Part model, mm, in its own coordinate system. Face numbers are marked on the shaded views. A direction names the side the tool comes from. Coordinates: 2 decimals unless noted, no trailing zeros. Write each loop counter-clockwise with the first axis right and the second up, starting at its lowest first coordinate (ties: lowest second). Pieces come first, ordered by that corner, then holes. Notation, with made-up numbers: (-29, 23) -> (2, 23) arc R34 ccw to (2, 57) -> close; hole circle Ø10 at (81, 79). An arc over 180 degrees is marked (long way). One line per question, with ' | ' between items. Start each with the question number.
Item 1: Pin check, flat tips, straight feed: pin 1 (4 mm diameter, centred on x = 27.5, z = 75.5, fed in from +Y); pin 2 (6 mm diameter, centred on x = 32.5, y = 32.5, fed in from -Z); pin 3 (1.5 mm diameter, centred on x = 27.5, z = 65, fed in from -Y). Stop position of each tip, or through.
Item 2: Saw through at C-C (z = 69). List the corners of the cut face in (x, y).
Item 3: 3-axis set-ups, long thin cutter, end or side, ignore diameter. For the marked faces 1, 2 and 3: which of +Z, -Z, +X, -X, +Y, -Y reach the whole face in a straight line?
Item 4: Saw through at A-A (y = 32.5). List the corners of the cut face in (x, z).
Item 5: Saw through at B-B (y = 3.5). List the corners of the cut face in (x, z).
Item 6: Probe probe 1 along Y at (x, z) = (-32.5, 7.5); probe 2 along Z at (x, y) = (12, -6.5). List the from-to ranges inside material, lowest first. Write a range as [from, to].
Item 7: Saw through at D-D (x = 0). List the corners of the cut face in (y, z).
from build123d import *

# Parameters (mm, degrees)
SKETCH_1_W          = 80
SKETCH_1_H          = 80
SKETCH_1_R          = 2.7
EXTRUDE_1_DEPTH     = 130
SKETCH_2_R          = 12.5
EXTRUDE_2_DEPTH     = 140
SKETCH_3_W          = 15
SKETCH_3_H          = 15
CUT_EXTRUDE_1_DEPTH = 120
FILLET_1_R          = 2
FILLET_3_R          = 10


with BuildPart() as part:
    # 草图1 → 凸台-拉伸1 (new body)
    with BuildSketch(Plane.XY):
        Rectangle(SKETCH_1_W, SKETCH_1_H)
        with Locations((-32.5, 32.5)):
            Circle(SKETCH_1_R, mode=Mode.SUBTRACT)
        with Locations((32.5, 32.5)):
            Circle(SKETCH_1_R, mode=Mode.SUBTRACT)
        with Locations((32.5, -32.5)):
            Circle(SKETCH_1_R, mode=Mode.SUBTRACT)
        with Locations((-32.5, -32.5)):
            Circle(SKETCH_1_R, mode=Mode.SUBTRACT)
    extrude(amount=EXTRUDE_1_DEPTH)

    # 草图2 → 凸台-拉伸2 (add)
    with BuildSketch(Plane(origin=(0, 0, 0), x_dir=(-1, 0, 0), z_dir=(0, 0, -1))):
        Circle(SKETCH_2_R)
    extrude(amount=EXTRUDE_2_DEPTH)

    # 草图3 → 切除-拉伸1 (cut)
    with BuildSketch(Plane.XY.offset(130)):
        with Locations((-32.5, 32.5)):
            Rectangle(SKETCH_3_W, SKETCH_3_H)
        with Locations((32.5, 32.5)):
            Rectangle(SKETCH_3_W, SKETCH_3_H)
        with Locations((32.5, -32.5)):
            Rectangle(SKETCH_3_W, SKETCH_3_H)
        with Locations((-32.5, -32.5)):
            Rectangle(SKETCH_3_W, SKETCH_3_H)
    extrude(amount=-CUT_EXTRUDE_1_DEPTH, mode=Mode.SUBTRACT)

    # 圆角1
    fillet_1_edges = [part.edges().sort_by_distance(p)[0] for p in [
        (40, -40, 5),
        (-40, -40, 5),
        (-40, 40, 5),
        (40, 40, 5),
    ]]
    fillet(fillet_1_edges, radius=FILLET_1_R)

    # 圆角3
    fillet_3_edges = [part.edges().sort_by_distance(p)[0] for p in [
        (-25, -40, 70),
        (-40, -25, 70),
        (40, -25, 70),
        (25, -40, 70),
        (25, 40, 70),
        (40, 25, 70),
        (-40, 25, 70),
        (-25, 40, 70),
    ]]
    fillet(fillet_3_edges, radius=FILLET_3_R)


solid = part.part
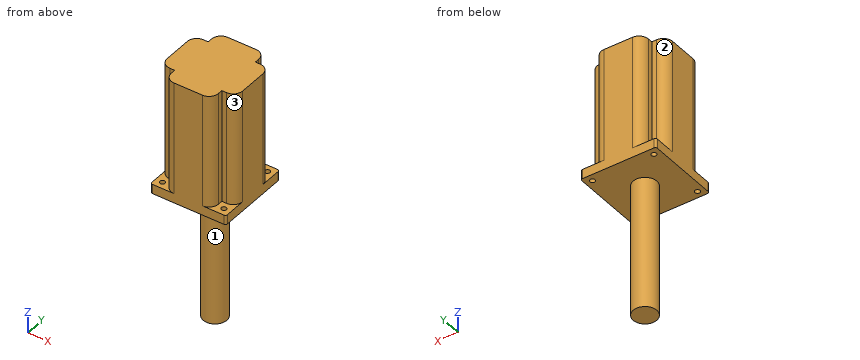
From the geometry:
1) pin 1: y = 25 | pin 2: z = 0 | pin 3: y = -25
2) outline: (-40, -15) arc R10 ccw to (-30, -25) -> (-25, -25) -> (-25, -30) arc R10 ccw to (-15, -40) -> (15, -40) arc R10 ccw to (25, -30) -> (25, -25) -> (30, -25) arc R10 ccw to (40, -15) -> (40, 15) arc R10 ccw to (30, 25) -> (25, 25) -> (25, 30) arc R10 ccw to (15, 40) -> (-15, 40) arc R10 ccw to (-25, 30) -> (-25, 25) -> (-30, 25) arc R10 ccw to (-40, 15) -> close
3) face 1: -Z | face 2: +Z, -X, +Y | face 3: +Z, +X, -Y
4) outline: (-40, 0) -> (-35.2, 0) -> (-35.2, 10) -> (-40, 10) -> close; (-29.8, 0) -> (29.8, 0) -> (29.8, 10) -> (24.68, 10) -> (24.68, 130) -> (-24.68, 130) -> (-24.68, 10) -> (-29.8, 10) -> close; (35.2, 0) -> (40, 0) -> (40, 10) -> (35.2, 10) -> close
5) outline: (-40, 0) -> (-12, 0) -> (-12, -140) -> (12, -140) -> (12, 0) -> (40, 0) -> (40, 130) -> (-40, 130) -> close
6) probe 1: [-40, -35.2], [-29.8, 29.8], [35.2, 40] | probe 2: [0, 130]
7) outline: (-40, 0) -> (-12.5, 0) -> (-12.5, -140) -> (12.5, -140) -> (12.5, 0) -> (40, 0) -> (40, 130) -> (-40, 130) -> close
